Verification items for the finished model (mm, model axes). Coordinates: 2 decimals unless noted, no trailing zeros. Write each loop counter-clockwise with the first axis right and the second up, starting at its lowest first coordinate (ties: lowest second). Pieces come first, ordered by that corner, then holes. Notation, with made-up numbers: (63.5, -12) -> (82.5, -12) arc R18 ccw to (82.5, 21) -> close; hole circle Ø7 at (-16, -4.75). An arc over 180 degrees is marked (long way). Write each question's results on one line, items separated by ' | '. Start each with the question number.
Autodesk Inventor part; units mm, degrees
ref_plane "YZ Plane" through (0, 0, 0) normal (1, 0, 0) x (0, 1, 0)
ref_plane "XZ Plane" through (0, 0, 0) normal (0, 1, 0) x (-1, 0, 0)
ref_plane "XY Plane" through (0, 0, 0) normal (0, 0, 1) x (1, 0, 0)
sketch "Sketch1" plane through (0, 0, 0) normal (0, 0, 1) x (1, 0, 0)
  line L0 (0, 177.8) -> (0, -177.8)
  line L1 (-66.675, 0) -> (288.925, 0)
  line L2 (15.875, -47.625) -> (-15.875, -47.625)
  line L3 (-15.875, -47.625) -> (-15.875, 47.625)
  line L4 (-15.875, 47.625) -> (15.875, 47.625)
  line L5 (15.875, 47.625) -> (15.875, -47.625)
  line L6 (0, 0) -> (0, 35.5411)
  circle A0 centre (71.6788, 0) radius 60.6679 construction
  circle A1 centre (71.6788, 0) radius 56.8579 construction
  circle A2 centre (71.6788, 0) radius 83.5279 construction
  line L7 (0, 47.625) -> (-15.875, 34.925) construction
  circle A3 centre (111.125, 0) radius 127
  point P0 (-10.795, 9.525)
  point P1 (-10.795, -9.525)
  point P2 (-6.985, 25.4)
  point P3 (-6.985, -25.4)
  dimension "d0" = 31.75
  dimension "d15" = 47.625
  dimension "d16" = 47.625
  dimension "d20" = 0
  dimension "d21" = 71.6788
  dimension "d22" = 121.3358
  dimension "d23" = 3.81
  dimension "d25" = 22.86
  dimension "d26" = 15.875
  dimension "d27" = 12.7
  dimension "d28" = 9.525
  dimension "d29" = 9.525
  dimension "d32" = 8.89
  dimension "d33" = 5.08
  dimension "d34" = 15.875
  dimension "d35" = 15.875
  dimension "d36" = 254
  dimension "d37" = 127
extrude "Extrusion1" add sketch "Sketch1" along normal blind 3.175 contours L1 A3 L4 L0 | L1 L5 L2 L0 | L0 L2 A3 L1 | L0 L4 L5 L1 | A3 L2 L3 | L3 L4 A3
hole "Hole1" at (-10.795, 9.525, 0) at (-10.795, -9.525, 0) at (-6.985, 25.4, 0) at (-6.985, -25.4, 0) direction (0, 0, 1) diameter 3.2512 end through all countersink diameter 6.35 countersink angle 90
fillet "Fillet1" radius 11.43 2 edges at (15.875, 47.625, 1.5875) (15.875, -47.625, 1.5875)
sketch "Sketch2" plane through (0, 0, 0) normal (0, 0, 1) x (1, 0, 0)
  circle A0 centre (111.125, 0) radius 127
  line L0 (4.445, 47.625) -> (-15.875, 47.625)
  line L1 (-15.875, -47.625) -> (4.445, -47.625)
  line L2 (-15.875, 47.625) -> (-15.875, -47.625)
  arc A1 (-6.6072, 47.625) -> (-6.6072, -47.625) centre (111.125, 0) ccw
  line L3 (-6.6072, 47.625) -> (-15.875, 47.625)
  line L4 (-15.875, 0) -> (-15.875, -47.625)
  line L5 (-15.875, -47.625) -> (-6.6072, -47.625)
  line L6 (-15.875, 47.625) -> (-15.875, 0)
  point P0 (0, 0)
extrude "Extrusion2" cut sketch "Sketch2" along normal blind 25.4 contours A0 L2 L0 | L1 L2 A0
fillet "Fillet2" radius 3.175 2 edges at (-6.6072, 47.625, 1.5875) (-6.6072, -47.625, 1.5875)
equation "\"d26\" = 0.5 * d0"
properties part number "J005322" material "STEEL, LOW CARBON (1008/1018/1020)"
1. Sectioned sample at B-B on y = -25.4. Record the cut outline in (x, z) (3 decimals).
2. Depth check by flat-ended pin: pin 1 Ø2 at (x, y) = (12.5, -15.5) entering from -Z; pin 2 Ø1.5 at (y, z) = (-15, 2) entering from -X. Enter the tip coordinate at first touch or a pass-through.
3. Sectioned sample at A-A on z = 0.65. Record the cut outline in (x, y) (3 decimals), plus the area to 3 significant figures.
4. Material ranges on probe 1 along X at (y, z) = (25.4, 2.2) (3 decimals); probe 2 along X at (y, z) = (10, 1.25) (3 decimals); probe 3 along Y at (x, z) = (8.5, 2.3), recorded low to high. Write a range as from..to.
5. Sectioned sample at C-C on x = 9. Record the cut outline in (y, z) (3 decimals).
Computed values:
1) outline: (-13.309, 0) -> (-10.16, 0) -> (-8.611, 1.549) -> (-8.611, 3.175) -> (-13.309, 3.175) -> close; (-5.359, 1.549) -> (-3.81, 0) -> (15.875, 0) -> (15.875, 3.175) -> (-5.359, 3.175) -> close
2) pin 1: stops at z = 0 | pin 2: stops at x = -15.07
3) outline: (-7.41, -45.59) arc R3.175 ccw to (-4.447, -47.625) -> (4.445, -47.625) arc R11.43 ccw to (15.875, -36.195) -> (15.875, 36.195) arc R11.43 ccw to (4.445, 47.625) -> (-4.447, 47.625) arc R3.175 ccw to (-7.41, 45.59) arc R127 ccw to start; hole circle Ø5.05 at (-10.795, -9.525); hole circle Ø5.05 at (-10.795, 9.525); hole circle Ø5.05 at (-6.985, -25.4); hole circle Ø5.05 at (-6.985, 25.4) | area: 2,600 mm^2
4) probe 1: x = -13.309..-8.611, -5.359..15.875 | probe 2: x = -15.481..-12.66, -8.93..15.875 | probe 3: y = -46.88..46.88
5) outline: (-46.678, 0) -> (46.678, 0) -> (46.678, 3.175) -> (-46.678, 3.175) -> close
